```python
from build123d import *

# Parameters (mm, degrees)
F0_W     = 838.2
F0_H     = 22.225
F1_DEPTH = 50.8
F3_DEPTH = 22.225
F4_W     = 31.75
F4_H     = 19.05
F5_DEPTH = 9.525


with BuildPart() as f1:
    # F0 (on Front) → F1 (new body)
    with BuildSketch(Plane.XZ):
        with Locations((419.1, 11.1125)):
            Rectangle(F0_W, F0_H)
    extrude(amount=F1_DEPTH)

    # F2 (on face) → F3 (cut)
    with BuildSketch(Plane.XZ.offset(50.8)):
        Polygon((405.591315, 22.225), (400.05, 0), (438.15, 0), (432.608685, 22.225), align=None)
        Polygon((792.941315, 22.225), (787.4, 0), (825.5, 0), (819.958685, 22.225), align=None)
        Polygon((12.7, 0), (50.8, 0), (45.258685, 22.225), (18.241315, 22.225), align=None)
    extrude(amount=-F3_DEPTH, mode=Mode.SUBTRACT)

    # F4 (on face) → F5 (cut)
    with BuildSketch(Plane.XY.offset(22.225)):
        with Locations((225.425, -9.525)):
            Rectangle(F4_W, F4_H)
        with Locations((606.425, -9.525)):
            Rectangle(F4_W, F4_H)
    extrude(amount=-F5_DEPTH, mode=Mode.SUBTRACT)


solid = f1.part
```
Could you check a few things on this model? Use its own coordinates, in mm. A direction names the side the tool comes from. Give positions to 0.01 mm unless a question says otherwise; leave off trailing zeros. Order: outer loops, then holes, each group sorted by start corner. A loop starts at its lowest first (then second) coordinate and runs counter-clockwise, first axis right, second up.
Q1. I'm going to push flat-ended pins straight in: P1, Ø6.5, axis at x = 805.5, z = 6, coming from the -Y side (3 decimals); P2, Ø10.5, axis at x = 217.5, z = 18, coming from the +Y side; P3, Ø9.5, axis at x = 599, y = -12.5, coming from the +Z side. Where does each tip first touch, or does it pass through?
Q2. Suppose I cut it at A-A, the plane y = -41. Write out the boundary of the cut face in (x, z) (3 decimals), and give its area (3 significant figures).
Q3. Suppose I cut it at B-B, the plane z = 6.75. Write out the boundary of the cut face in (x, y) (3 decimals), and give its area (3 significant figures).
Q4. We'd pull the mould along X, two halves only. Please class faces 3 (the flat face through (225, -9, 12.7)), 4 (the flat face through (831, -50.8, 11)), 5 (the flat face through (838.2, -25, 11)): +X half, -X half, draft (parallel to the pull), parting line (faces both ways), or undercut.
Q5. If I drill on line 1 along X through (y, z) = (-9.5, 21.25); line 2 along X through (y, z) = (-39.5, 15); line 3 along X through (y, z) = (-40, 18.5), over which ranges is the centre line in solid material (lowest first)?
Q6. Suppose I cut it at C-C, the plane y = -10.5. Write out the boundary of the cut face in (x, z) (3 decimals), and give its area (3 significant figures).
Q7. For faces 1 (the flat face through (223, -50.8, 11)), 2 (the flat face through (15.51, -39.84, 11.27)), which set-ups out of +Z, -Z, +X, -X, +Y, -Y let a thin tool reach every point of the face, with its end or its side?
Solution:
1. P1: stops at y = -28.575
1. P2: stops at y = -19.05
1. P3: stops at z = 12.7
2. outline: (0, 0) - (12.7, 0) - (18.241, 22.225) - (0, 22.225) - close; (45.259, 22.225) - (50.8, 0) - (400.05, 0) - (405.591, 22.225) - close; (432.609, 22.225) - (438.15, 0) - (787.4, 0) - (792.941, 22.225) - close; (819.959, 22.225) - (825.5, 0) - (838.2, 0) - (838.2, 22.225) - close
2. area: 16,500 mm2
3. outline: (0, -50.8) - (14.383, -50.8) - (14.383, -28.575) - (49.117, -28.575) - (49.117, -50.8) - (401.733, -50.8) - (401.733, -28.575) - (436.467, -28.575) - (436.467, -50.8) - (789.083, -50.8) - (789.083, -28.575) - (823.817, -28.575) - (823.817, -50.8) - (838.2, -50.8) - (838.2, 0) - (0, 0) - close
3. area: 40,300 mm2
4. face 3: undercut
4. face 4: draft
4. face 5: +X half
5. line 1: x = 0 to 209.55, 241.3 to 590.55, 622.3 to 838.2
5. line 2: x = 0 to 16.44, 47.06 to 403.79, 434.41 to 791.14, 821.76 to 838.2
5. line 3: x = 0 to 17.31, 46.19 to 404.66, 433.54 to 792.01, 820.89 to 838.2
6. outline: (0, 0) - (838.2, 0) - (838.2, 22.225) - (622.3, 22.225) - (622.3, 12.7) - (590.55, 12.7) - (590.55, 22.225) - (241.3, 22.225) - (241.3, 12.7) - (209.55, 12.7) - (209.55, 22.225) - (0, 22.225) - close
6. area: 18,000 mm2
7. face 1: +Z, -Z, +X, -X, -Y
7. face 2: -Z, -Y
